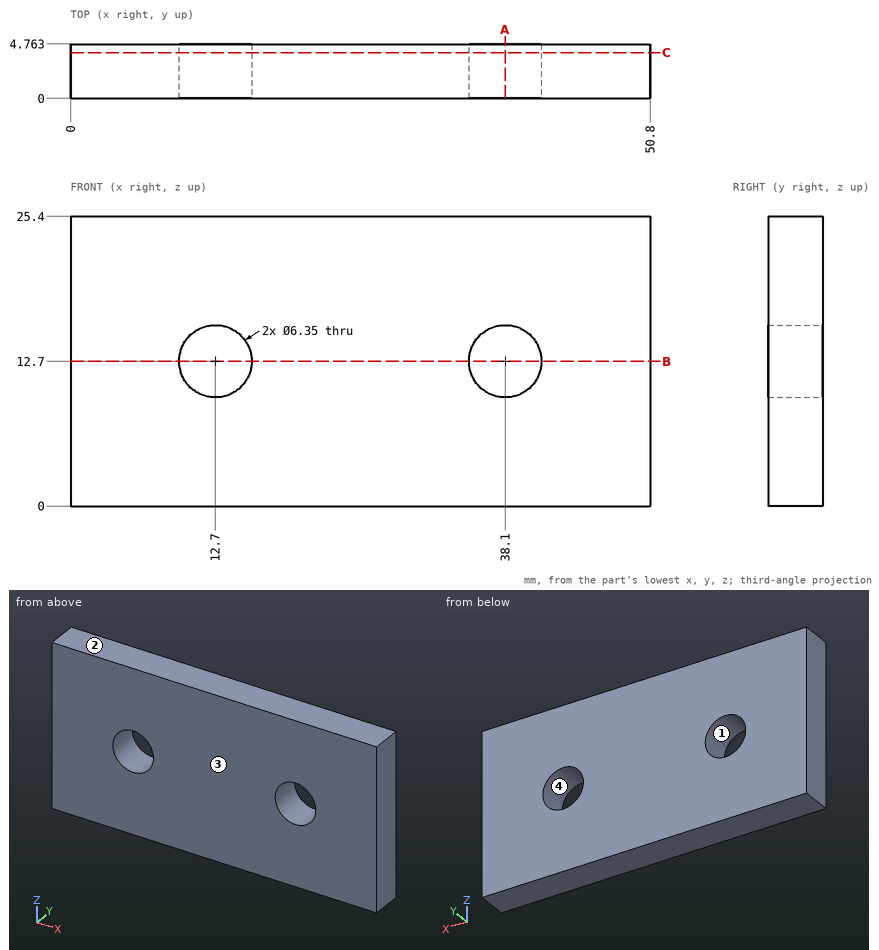
Study the drawing (mm; zero at the part's minimum x, y, z) and answer. Round coordinates to 2 decimals unless told otherwise and drop trailing zeros. Write each loop counter-clockwise with the first axis right and the second up, starting at its lowest first coordinate (ties: lowest second). Pieces come first, ordered by that corner, then holes. Notation, with made-up numbers: (-5.75, 14.25) - (51.25, 14.25) arc R24 ccw to (51.25, 29.25) - close; hole circle Ø6 at (55, 29). An arc over 180 degrees is marked (long way). Use CSV: the item, a comma, the result in double quotes.
Q1. Find section A-A, the plane x = 38.1. Write down the section's boundary in (y, z) (1 decimal).
Values:
outline,"(0, 0) - (4.8, 0) - (4.8, 9.5) - (0, 9.5) - close; (0, 15.9) - (4.8, 15.9) - (4.8, 25.4) - (0, 25.4) - close"
Q2. Straight lines are drawn through the part: line 1 along X through (y, z) = (3, 12.7) (1 decimal); line 2 along Z through (x, y) = (12.7, 2.4) (1 decimal); line 3 along Z through (x, y) = (12, 2.45). For each, find the intervals that lie inside material, in ascending order.
Values:
line 1,"x = 0 to 9.5, 15.9 to 34.9, 41.3 to 50.8"
line 2,"z = 0 to 9.5, 15.9 to 25.4"
line 3,"z = 0 to 9.6, 15.8 to 25.4"
Q3. Find section B-B, the plane z = 12.7. Write down the section's boundary in (x, y) (1 decimal).
Values:
outline,"(0, 0) - (9.5, 0) - (9.5, 4.8) - (0, 4.8) - close; (15.9, 0) - (34.9, 0) - (34.9, 4.8) - (15.9, 4.8) - close; (41.3, 0) - (50.8, 0) - (50.8, 4.8) - (41.3, 4.8) - close"
Q4. Each of these flat-tipped pins is pushed along its axis until it touches: pin 1 Ø5 at (x, z) = (12.7, 12.7) entering from +Y; pin 2 Ø1.5 at (x, y) = (44.5, 2.5) entering from -Z. Where does it stop, or does it pass through?
Values:
pin 1,"passes through"
pin 2,"stops at z = 0"
Q5. Determine the mould class of the marked faces 1, 2, 3 and 4 for opening direction Z: +Z half, -Z half, draft (parallel to the pull), parting line (faces both ways), or undercut.
Values:
face 1,"undercut"
face 2,"+Z half"
face 3,"draft"
face 4,"undercut"
Q6. Find section C-C, the plane y = 4. Count the separate pieces of the cut face and the enclosed holes in it, then the cut area to 3 significant figures.
Values:
separate pieces,"1"
enclosed holes,"2"
area,"1,230 mm²"
